```python
from build123d import *

# Parameters (mm, degrees)
F0_W     = 45.113686
F0_H     = 60.767936
F0_R     = 12.848054
F0_R_2   = 5.3975
F1_DEPTH = 6.35
F2_DEPTH = 3.175


with BuildPart() as f1:
    # F0 (on Top) → F1 (new body)
    with BuildSketch(Plane.XY):
        Rectangle(F0_W, F0_H)
        Circle(F0_R, mode=Mode.SUBTRACT)
        Circle(F0_R)
        Circle(F0_R_2, mode=Mode.SUBTRACT)
    extrude(amount=-F1_DEPTH)

    # F0 (on Top) → F2 (join)
    with BuildSketch(Plane.XY):
        Circle(F0_R)
        Circle(F0_R_2, mode=Mode.SUBTRACT)
    extrude(amount=F2_DEPTH)


solid = f1.part
```
Can you work these out from the model? Positions are in its coordinate system, mm. Coordinates: 2 decimals unless noted, no trailing zeros. Write each loop counter-clockwise with the first axis right and the second up, starting at its lowest first coordinate (ties: lowest second). Pieces come first, ordered by that corner, then holes. Notation, with made-up numbers: M -20.5,9.5 L 13.5,9.5 A34 cw 13.5,46.5 Z; hole C 55.25,41.5 d6. An arc over 180 degrees is marked long. Answer as CSV lines item,"result".
Item 1: Imagine slicing it at D-D on y = 17. List the corners of the cut face in (x, z) for me.
Geometry results:
outline,"M -22.56,-6.35 L 22.56,-6.35 L 22.56,0 L -22.56,0 Z"
Item 2: We'd pull the mould along Y, two halves only. Please class faces 1 (the flat face through (0, -30.384, -3)), 2 (the cylindrical face through (-3.978, 3.648, -1.654)), 3 (the cylindrical face through (12.255, 3.859, 1.565)), 4 (the flat face through (0, -13, 0)): +Y half, -Y half, draft (parallel to the pull), parting line (faces both ways), or undercut.
Geometry results:
face 1,"-Y half"
face 2,"undercut"
face 3,"parting line"
face 4,"draft"
Item 3: Imagine slicing it at C-C on z = -2. List the corners of the cut face in (x, y) for me (1 decimal).
Geometry results:
outline,"M -22.6,-30.4 L 22.6,-30.4 L 22.6,30.4 L -22.6,30.4 Z; hole C 0,0 d10.8"
Item 4: I'm going to push a flat-ended pin straight in: P1, Ø9.5, axis at x = 0, y = 0, coming from the +Z side. Where does the tip first touch, or does it pass through?
Geometry results:
P1,"passes through"
Item 5: Please list where these lines run through material, in increasing order: line 1 along Y through (x, z) = (0, -3); line 2 along Z through (x, y) = (-10, 23); line 3 along Y through (x, z) = (-3, 2.5).
Geometry results:
line 1,"y = -30.38 to -5.4, 5.4 to 30.38"
line 2,"z = -6.35 to 0"
line 3,"y = -12.49 to -4.49, 4.49 to 12.49"
